Source: three-view drawing plus pictorial views. Frame: mm from the lowest corner of the part. A direction names the side the tool comes from. Coordinates: 2 decimals unless noted, no trailing zeros. Write each loop counter-clockwise with the first axis right and the second up, starting at its lowest first coordinate (ties: lowest second). Pieces come first, ordered by that corner, then holes.
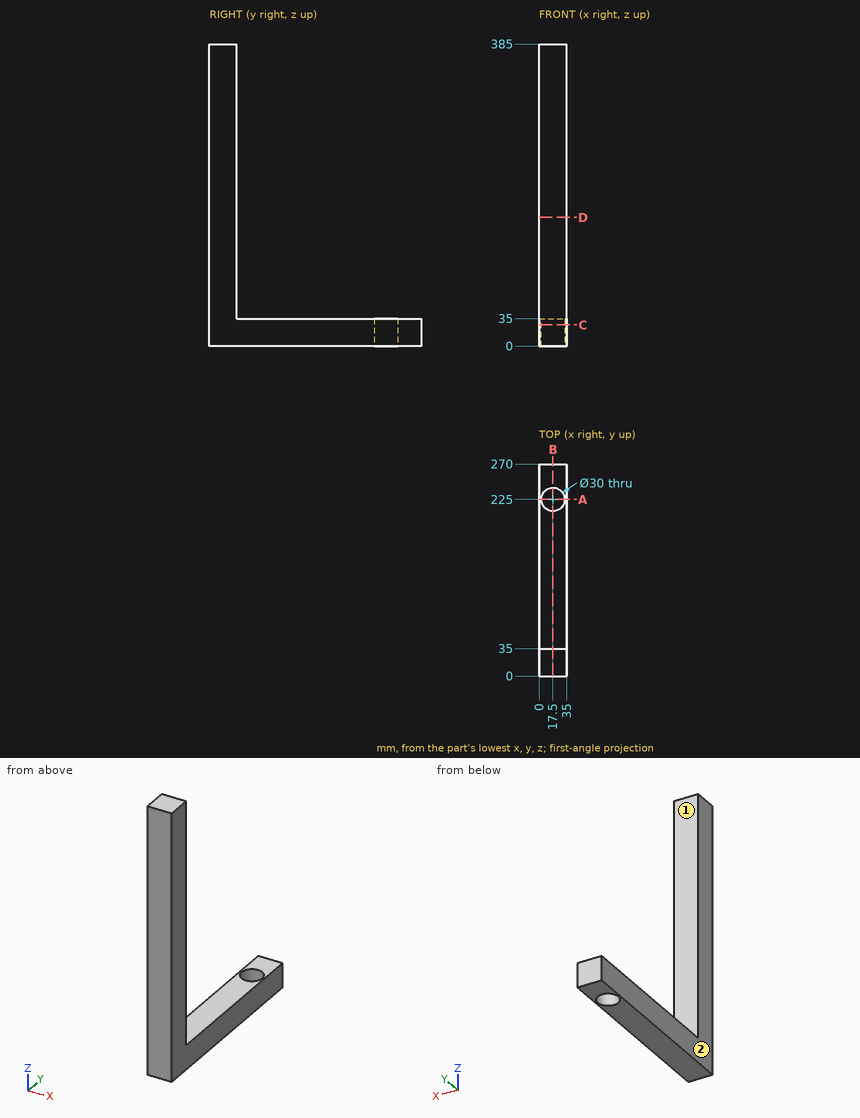
Item 1: Section query D-D, the plane z = 164. Return loops of the section in (x, y), then the cut area to 4 significant figures.
Item 2: Pin query (flat end, axial travel): pin 1 Ø10 at (x, z) = (13, 166) entering from +Y; pin 2 Ø10.5 at (x, y) = (15, 168) entering from +Z. Return the tip coordinate at first contact, or that it passes through.
Item 3: Section query A-A, the plane y = 225. Return loops of the section in (x, z), then the cut area to 3 significant figures.
Item 4: Section query B-B, the plane x = 17.5. Return loops of the section in (y, z).
Item 5: Access query for the marked faces 1 and 2. Directions: +Z, -Z, +X, -X, +Y, -Y. A direction counts if a zero-diameter tool reaches every point of the face in a straight line with its end or side. Return the directions, or none.
Item 6: Material intervals for line 1 (Y direction, x = 17.5, z = 26.5); line 2 (Y direction, x = 2.5, z = 329), sorted ascending.
Item 7: Section query C-C, the plane z = 27. Return loops of the section in (x, y), then the cut area to 3 significant figures.
The answers:
1. outline: (0, 0) - (35, 0) - (35, 35) - (0, 35) - close
1. area: 1,225 mm2
2. pin 1: stops at y = 35
2. pin 2: stops at z = 35
3. outline: (0, 0) - (2.5, 0) - (2.5, 35) - (0, 35) - close; (32.5, 0) - (35, 0) - (35, 35) - (32.5, 35) - close
3. area: 175 mm2
4. outline: (0, 0) - (210, 0) - (210, 35) - (35, 35) - (35, 385) - (0, 385) - close; (240, 0) - (270, 0) - (270, 35) - (240, 35) - close
5. face 1: +Z, +X, -X, +Y
5. face 2: +Z, -Z, -X, +Y, -Y
6. line 1: y = 0 to 210, 240 to 270
6. line 2: y = 0 to 35
7. outline: (0, 0) - (35, 0) - (35, 270) - (0, 270) - close; hole circle Ø30 at (17.5, 225)
7. area: 8,740 mm2
